Could you check a few things on this model? Use its own coordinates, in mm. A direction names the side the tool comes from. Coordinates: 2 decimals unless noted, no trailing zeros. Loops run counter-clockwise (first coordinate to the right, second up) from the corner with the lowest first, then second, coordinate; pieces in that order, holes last. Notation, with made-up numbers: (6.5, 19.25) - (44.5, 19.25) arc R24 ccw to (44.5, 43.25) - close; hole circle Ø3 at (26.25, 16). An arc over 180 degrees is marked (long way). Put each result on its own line as item: value. Start each with the question number.
Autodesk Inventor part; units mm, degrees
ref_plane "YZ Plane" through (0, 0, 0) normal (1, 0, 0) x (0, 1, 0)
ref_plane "XZ Plane" through (0, 0, 0) normal (0, 1, 0) x (-1, 0, 0)
ref_plane "XY Plane" through (0, 0, 0) normal (0, 0, 1) x (1, 0, 0)
sketch "Sketch1" plane through (0, 0, 0) normal (1, 0, 0) x (0, 1, 0)
  line L0 (9.6754, 10.4121) -> (-4.2246, 10.4121)
  line L1 (-4.2246, 10.4121) -> (-4.2246, -12.5879)
  line L2 (-4.2246, -12.5879) -> (9.6754, -12.5879)
  line L3 (9.6754, -12.5879) -> (9.6754, 10.4121)
  line L4 (9.6754, -1.0879) -> (8.0754, -1.0879) construction
  line L5 (8.0754, -1.0879) -> (8.0754, -8.0879) construction
  line L6 (8.0754, -8.0879) -> (8.0754, 5.9121) construction
  line L7 (8.0754, 5.9121) -> (6.4254, 5.9121) construction
  circle A0 centre (6.4254, 5.9121) radius 1.65
  circle A1 centre (6.4254, -8.0879) radius 1.65
  point P0 (0, 0)
  dimension "d0" = 13.9
  dimension "d1" = 23
  dimension "d7" = 1.6
  dimension "d8" = 7
  dimension "d9" = 90
  dimension "d10" = 14
  dimension "d11" = 1.65
  dimension "d12" = 3.3
  dimension "d13" = 3.3
extrude "Extrusion1" add sketch "Sketch1" along normal blind 2.87
sketch "Sketch2" plane through (2.87, 0, 0) normal (1, 0, 0) x (0, 0, -1)
  line L0 (12.5879, -4.2246) -> (12.5879, 9.6754)
  line L1 (-10.4121, -4.2246) -> (12.5879, -4.2246)
  line L2 (12.5879, -4.2246) -> (12.5879, 3.2154)
  line L3 (12.5879, 3.2154) -> (-10.4121, 3.2154)
  line L4 (-10.4121, 3.2154) -> (-10.4121, -4.2246)
  point P0 (0, 0)
  dimension "d4" = 7.44
extrude "Extrusion2" add sketch "Sketch2" along normal blind 3
properties part number "reed_switch"
(1) I want a section at A-A on z = 4.5. List the corners of the cut face in (x, y) for me, and give its area (3 significant figures).
(2) I want a section at B-B on y = 5.5. List the corners of the cut face in (x, z) for me, and give its area (3 significant figures).
(3) For pin 1 Ø5.5 at (y, z) = (6.43, -8.09) entering from +X; pin 2 Ø2.5 at (x, z) = (5, -3) entering from +Y; pin 3 Ø2 at (y, z) = (6.43, 5.91) entering from +X, each with a flat end and sliding along its axis, tell me the tip position at first contact or that it passes through.
(4) I need wall thicknesses on L1, parallel to X at y = 6.75, z = -5; L2, parallel to Y at x = 3.1, z = -1.25; L3, parallel to Z at x = 1.3, y = 6.75. Which ranges of each line are inside material? Lowest first, please. Write a range as [from, to].
(5) If we mould it in two halves opening along Z, with no side actions, what happens to faces 3 (the cylindrical face through (1.41, 5.12, -7.08)), 4 (the flat face through (2, 1, 10.412)), 5 (the flat face through (4, 3.215, -1))? For each: pulls with the +Z half, pulls with the -Z half, needs draft (parallel to the pull), parting line crosses it, or undercut.
(6) I want a section at D-D on x = 2.25. List the corners of the cut face in (y, z) for me.
(7) Which directions (+Z, -Z, +X, -X, +Y, -Y) give clear straight access to the entire face, cutting with the end or side of a thin tool? Please do faces 1 (the flat face through (0, 3, -1)), 2 (the flat face through (2.87, 6, -1)).
(8) I want a section at C-C on z = -4. List the corners of the cut face in (x, y) for me, and give its area (3 significant figures).
Answer sheet:
1. outline: (0, -4.22) - (5.87, -4.22) - (5.87, 3.22) - (2.87, 3.22) - (2.87, 5.57) - (0, 5.57) - close; (0, 7.28) - (2.87, 7.28) - (2.87, 9.68) - (0, 9.68) - close
1. area: 57.3 mm^2
2. outline: (0, -12.59) - (2.87, -12.59) - (2.87, -9.45) - (0, -9.45) - close; (0, -6.72) - (2.87, -6.72) - (2.87, 4.55) - (0, 4.55) - close; (0, 7.28) - (2.87, 7.28) - (2.87, 10.41) - (0, 10.41) - close
2. area: 50.3 mm^2
3. pin 1: stops at x = 2.87
3. pin 2: stops at y = 3.22
3. pin 3: passes through
4. L1: x = [0, 2.87]
4. L2: y = [-4.22, 3.22]
4. L3: z = [-12.59, -9.71], [-6.47, 4.29], [7.53, 10.41]
5. face 3: undercut
5. face 4: pulls with the +Z half
5. face 5: needs draft
6. outline: (-4.22, -12.59) - (9.68, -12.59) - (9.68, 10.41) - (-4.22, 10.41) - close; hole circle Ø3.3 at (6.43, -8.09); hole circle Ø3.3 at (6.43, 5.91)
7. face 1: +Z, -Z, -X, +Y, -Y
7. face 2: +Z, -Z, +X, +Y
8. outline: (0, -4.22) - (5.87, -4.22) - (5.87, 3.22) - (2.87, 3.22) - (2.87, 9.68) - (0, 9.68) - close
8. area: 62.2 mm^2
